Build history of the part. All positions in model axes, mm. A direction names the side the tool comes from. Round coordinates to 2 decimals unless told otherwise and drop trailing zeros. Order: outer loops, then holes, each group sorted by start corner. A loop starts at its lowest first (then second) coordinate and runs counter-clockwise, first axis right, second up. Notation, with made-up numbers: (10.25, 52) -> (22.25, 52) arc R17 ccw to (22.25, 75) -> close; hole circle Ø8 at (-31.75, 33.5). An arc over 180 degrees is marked (long way). Answer as a JSON object with one key per item and string values.
from build123d import *

# Parameters (mm, degrees)
SKETCH_W      = 30
SKETCH_H      = 35
PAD_DEPTH     = 3
SKETCH001_R   = 10
SKETCH001_R_2 = 8.5
PAD001_DEPTH  = 10
PAD002_DEPTH  = 7


with BuildPart() as part:
    # Sketch → Pad (new body)
    with BuildSketch(Plane.XY):
        Rectangle(SKETCH_W, SKETCH_H)
    extrude(amount=-PAD_DEPTH)

    # Sketch001 → Pad001 (join)
    with BuildSketch(Plane.XY):
        with Locations((0, -5)):
            Circle(SKETCH001_R)
        with Locations((0, -5)):
            Circle(SKETCH001_R_2, mode=Mode.SUBTRACT)
    extrude(amount=PAD001_DEPTH)

    # Sketch002 → Pad002 (join)
    with BuildSketch(Plane.XY):
        with BuildLine():
            ThreePointArc((-7, 14.5), (-10.5, 11), (-7, 7.5))
            Line((-7, 7.5), (7, 7.5))
            ThreePointArc((7, 7.5), (10.5, 11), (7, 14.5))
            Line((-7, 14.5), (7, 14.5))
        make_face()
        with BuildLine():
            ThreePointArc((-7, 13.5), (-9.5, 11), (-7, 8.5))
            Line((-7, 8.5), (7, 8.5))
            ThreePointArc((7, 8.5), (9.5, 11), (7, 13.5))
            Line((-7, 13.5), (7, 13.5))
        make_face(mode=Mode.SUBTRACT)
    extrude(amount=PAD002_DEPTH)


solid = part.part
1) Which spindle directions (+Z, -Z, +X, -X, +Y, -Y) get a long thin tool onto all of the face, cutting with end or side? Do faces 1 (the face through (10.5, 10.9, 3.5)), 2 (the face through (0, 7.5, 3)), 3 (the face through (0, 14.5, 3)), 4 (the face through (0, 11, 0)). Say none if no direction does.
Checked values:
{"face 1": "+Z, +X", "face 2": "+Z, +X, -X", "face 3": "+Z, +X, -X, +Y", "face 4": "+Z"}
2) Probe L1, parallel to Y at x = 0, z = 3.25; L2, parallel to X at y = 11, z = 1.5; L3, parallel to Y at x = 0, z = 8. List the from-to ranges inside material, lowest first. Write a range as from..to.
Checked values:
{"L1": "y = -15..-13.5, 3.5..5, 7.5..8.5, 13.5..14.5", "L2": "x = -10.5..-9.5, 9.5..10.5", "L3": "y = -15..-13.5, 3.5..5"}
3) Pull direction Y, two halves, no side cores. Call faces 5 (the face through (-10.5, 11.1, 3.5)), 6 (the face through (0, 8, 7)), 7 (the face through (0, -17.5, -1)): pulls with the +Y half, pulls with the -Y half, needs draft (parallel to the pull), parting line crosses it, or undercut.
Checked values:
{"face 5": "undercut", "face 6": "needs draft", "face 7": "pulls with the -Y half"}
4) Cut at B-B, the plane y = 11. Give the cut face in (x, z).
Checked values:
{"outline": "(-15, -3) -> (15, -3) -> (15, 0) -> (10.5, 0) -> (10.5, 7) -> (9.5, 7) -> (9.5, 0) -> (-9.5, 0) -> (-9.5, 7) -> (-10.5, 7) -> (-10.5, 0) -> (-15, 0) -> close"}
5) Cut at C-C, the plane x = 0. Give the cut face in (y, z), plus the area to 3 significant figures.
Checked values:
{"outline": "(-17.5, -3) -> (17.5, -3) -> (17.5, 0) -> (14.5, 0) -> (14.5, 7) -> (13.5, 7) -> (13.5, 0) -> (8.5, 0) -> (8.5, 7) -> (7.5, 7) -> (7.5, 0) -> (5, 0) -> (5, 10) -> (3.5, 10) -> (3.5, 0) -> (-13.5, 0) -> (-13.5, 10) -> (-15, 10) -> (-15, 0) -> (-17.5, 0) -> close", "area": "149 mm²"}
6) Cut at D-D, the plane z = 9.25. Give the cut face in (x, y), plus the area to 3 significant figures.
Checked values:
{"outline": "circle Ø20 at (0, -5); hole circle Ø17 at (0, -5)", "area": "87.2 mm²"}
7) Flat gauge pins, fed straight in: pin 1 Ø3 at (y, z) = (-8.5, 7.5) entering from +X; pin 2 Ø3 at (x, z) = (6.5, 4) entering from +Y; pin 3 Ø1 at (x, z) = (-6.5, 8) entering from -Y; pin 4 Ø4 at (y, z) = (6, 1) entering from -X. Where does each tip first touch, or does it go through?
Checked values:
{"pin 1": "stops at x = 9.8", "pin 2": "stops at y = 14.5", "pin 3": "stops at y = -13", "pin 4": "stops at x = -15"}
8) Cut at A-A, the plane z = 1.75. Give the cut face in (x, y), plus the area to 3 significant figures.
Checked values:
{"outline": "circle Ø20 at (0, -5); (-7, 7.5) -> (7, 7.5) arc R3.5 ccw to (7, 14.5) -> (-7, 14.5) arc R3.5 ccw to start; hole circle Ø17 at (0, -5); hole (-7, 8.5) -> (7, 8.5) arc R2.5 ccw to (7, 13.5) -> (-7, 13.5) arc R2.5 ccw to start", "area": "134 mm²"}
